Check sheet for the modelled part. Datum: model origin and axes. Units: mm. Coordinates: 2 decimals unless noted, no trailing zeros. Write each loop counter-clockwise with the first axis right and the second up, starting at its lowest first coordinate (ties: lowest second). Pieces come first, ordered by that corner, then holes. Notation, with made-up numbers: (-9.75, 48.25) - (40.25, 48.25) arc R11 ccw to (40.25, 63.25) - close; hole circle Ø2 at (17.25, 80.5). An arc over 180 degrees is marked (long way). Use one line per item in the form item = value. Start each with the question number.
1. Scan lines: line 1 along X through (y, z) = (-2.7, 17); line 2 along X through (y, z) = (-2.25, 11.5); line 3 along X through (y, z) = (-4.85, 4). Record each from-to range of solid material in increasing order.
2. Cross-section at D-D on x = 27. Record the boundary of the cut face in (y, z).
3. Cross-section at B-B on y = -3.95. Give the number of separate pieces and of enclosed holes in the cut face, then the cut area to 3 significant figures.
4. Cross-section at C-C on x = 79.5. Record the boundary of the cut face in (y, z).
5. Go/stop test with flat-tipped pins: pin 1 Ø2.5 at (y, z) = (-4.5, 20) entering from -X; pin 2 Ø1.5 at (y, z) = (-5, 26) entering from +X; pin 3 Ø2.5 at (y, z) = (-4.5, 22.5) entering from -X. Record where each tip stops, or that it passes through.
6. Cross-section at A-A on z = 20. Record the boundary of the cut face in (x, y), then the cut area to 3 significant figures.
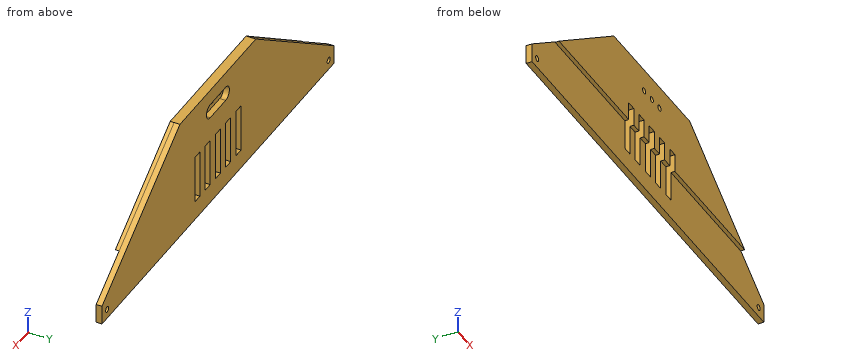
```python
from build123d import *

# Parameters (mm, degrees)
PAD_DEPTH       = 5
SKETCH001_R     = 1.5
POCKET_DEPTH    = 5.001
SKETCH002_R     = 1.5
PAD001_DEPTH    = 2
POCKET001_DEPTH = 5
SKETCH004_W     = 5
SKETCH004_H     = 25
POCKET002_DEPTH = 7.001
SKETCH005_W     = 243.085243
SKETCH005_H     = 32.517023
POCKET003_DEPTH = 2
SKETCH006_W     = 324.151733
SKETCH006_H     = 177.952698
POCKET004_DEPTH = 2


with BuildPart() as part:
    # Sketch → Pad (new body)
    with BuildSketch(Plane.XZ):
        Polygon((-37, 63.25), (37, 63.25), (113, 10), (113, 0), (-113, 0), (-113, 10), align=None)
    extrude(amount=PAD_DEPTH)

    # Sketch001 (on Face8 of Pad) → Pocket (cut, through all)
    with BuildSketch(Plane.XZ.offset(5)):
        with Locations((-108, 5)):
            Circle(SKETCH001_R)
        with Locations((108, 5)):
            Circle(SKETCH001_R)
        with Locations((-7.5, 51.5)):
            Circle(SKETCH001_R)
        with Locations((0, 51.5)):
            Circle(SKETCH001_R)
        with Locations((7.5, 51.5)):
            Circle(SKETCH001_R)
    extrude(amount=-POCKET_DEPTH, mode=Mode.SUBTRACT)

    # Sketch002 (on Face5 of Pocket) → Pad001 (join)
    with BuildSketch(Plane.XZ.offset(5)):
        Polygon((-37, 63.25), (37, 63.25), (104.655786, 15.55), (-104.655786, 15.55), align=None)
        with Locations((-7.5, 51.5)):
            Circle(SKETCH002_R, mode=Mode.SUBTRACT)
        with Locations((0, 51.5)):
            Circle(SKETCH002_R, mode=Mode.SUBTRACT)
        with Locations((7.5, 51.5)):
            Circle(SKETCH002_R, mode=Mode.SUBTRACT)
    extrude(amount=PAD001_DEPTH)

    # Sketch003 (on Face4 of Pad001) → Pocket001 (cut)
    with BuildSketch(Plane(origin=(0, 0, 0), x_dir=(1, 0, 0), z_dir=(0, 1, 0))):
        with BuildLine():
            ThreePointArc((-7.5, -47.798047), (-11.201953, -51.5), (-7.5, -55.201953))
            Line((-7.5, -55.201953), (7.5, -55.201953))
            ThreePointArc((7.5, -55.201953), (11.201953, -51.5), (7.5, -47.798047))
            Line((7.5, -47.798047), (-7.5, -47.798047))
        make_face()
    extrude(amount=-POCKET001_DEPTH, mode=Mode.SUBTRACT)

    # Sketch004 (on Face4 of Pocket001) → Pocket002 (cut, through all)
    with BuildSketch(Plane(origin=(0, 0, 0), x_dir=(1, 0, 0), z_dir=(0, 1, 0))):
        with Locations((-20, -22.5)):
            Rectangle(SKETCH004_W, SKETCH004_H)
        with Locations((0, -22.5)):
            Rectangle(SKETCH004_W, SKETCH004_H)
        with Locations((10, -22.5)):
            Rectangle(SKETCH004_W, SKETCH004_H)
        with Locations((20, -22.5)):
            Rectangle(SKETCH004_W, SKETCH004_H)
        with Locations((-10, -22.5)):
            Rectangle(SKETCH004_W, SKETCH004_H)
    extrude(amount=-POCKET002_DEPTH, mode=Mode.SUBTRACT)

    # Sketch005 (on Face38 of Pocket002) → Pocket003 (cut)
    with BuildSketch(Plane.XZ.offset(7)):
        with Locations((0.109928, 9.291488)):
            Rectangle(SKETCH005_W, SKETCH005_H)
    extrude(amount=-POCKET003_DEPTH, mode=Mode.SUBTRACT)

    # Sketch006 (on Face4 of Pocket003) → Pocket004 (cut)
    with BuildSketch(Plane(origin=(0, 0, 0), x_dir=(1, 0, 0), z_dir=(0, 1, 0))):
        with Locations((27.792465, -47.893646)):
            Rectangle(SKETCH006_W, SKETCH006_H)
    extrude(amount=-POCKET004_DEPTH, mode=Mode.SUBTRACT)


solid = part.part
```
Final values:
q1.line_1 = -103.01 to -22.5, -17.5 to -12.5, -7.5 to -2.5, 2.5 to 7.5, 12.5 to 17.5, 22.5 to 103.01
q1.line_2 = -110.86 to -22.5, -17.5 to -12.5, -7.5 to -2.5, 2.5 to 7.5, 12.5 to 17.5, 22.5 to 110.86
q1.line_3 = -113 to -109.12, -106.88 to 106.88, 109.12 to 113
q2.outline = (-7, 25.55) - (-5, 25.55) - (-5, 0) - (-2, 0) - (-2, 63.25) - (-7, 63.25) - close
q3.separate_pieces = 1
q3.enclosed_holes = 8
q3.area = 9,450 mm²
q4.outline = (-7, 25.55) - (-5, 25.55) - (-5, 0) - (-2, 0) - (-2, 33.47) - (-5, 33.47) - (-5, 33.29) - (-7, 33.29) - close
q5.pin_1 = -100.51
q5.pin_2 = 91.23
q5.pin_3 = -96.94
q6.outline = (-98.73, -5) - (-22.5, -5) - (-22.5, -2) - (-98.73, -2) - close; (-17.5, -5) - (-12.5, -5) - (-12.5, -2) - (-17.5, -2) - close; (-7.5, -5) - (-2.5, -5) - (-2.5, -2) - (-7.5, -2) - close; (2.5, -5) - (7.5, -5) - (7.5, -2) - (2.5, -2) - close; (12.5, -5) - (17.5, -5) - (17.5, -2) - (12.5, -2) - close; (22.5, -5) - (98.73, -5) - (98.73, -2) - (22.5, -2) - close
q6.area = 517 mm²
